from build123d import *

# Parameters (mm, degrees)
EXTRUDE_1_DEPTH     = 4.6
SKETCH_1_R          = 2.625
SKETCH_1_W          = 40.4
SKETCH_1_H          = 4.6
CUT_EXTRUDE_1_DEPTH = 4.6
FILLET_1_R          = 5
FILLET_2_R          = 4


with BuildPart() as part:
    # 草图3 → 凸台-拉伸1 (new body)
    with BuildSketch(Plane(origin=(0, 0, 0), x_dir=(1, 0, 0), z_dir=(0, 1, 0))):
        Polygon((-40, 28), (-60, 28), (-60, -28), (-40, -28), (18.5, -28), (18.5, -36), (45, -36), (45, -28), (45, 28), (45, 36), (18.5, 36), (18.5, 28), align=None)
    extrude(amount=EXTRUDE_1_DEPTH)

    # 草图1 → 切除-拉伸1 (cut)
    with BuildSketch(Plane(origin=(0, 0, 0), x_dir=(1, 0, 0), z_dir=(0, 1, 0))):
        with Locations(Location((-31.75, 20.6375, 0), (0, 0, 270))):
            Circle(SKETCH_1_R)
        with Locations(Location((31.75, 20.6375, 0), (0, 0, 90))):
            Circle(SKETCH_1_R)
        with Locations(Location((31.75, -20.6375, 0), (0, 0, 270))):
            Circle(SKETCH_1_R)
        with Locations(Location((-31.75, -20.6375, 0), (0, 0, 90))):
            Circle(SKETCH_1_R)
        with Locations((-28, -10.4375)):
            Rectangle(SKETCH_1_W, SKETCH_1_H)
        with Locations((-28, 10.4375)):
            Rectangle(SKETCH_1_W, SKETCH_1_H)
        Polygon((-22.25, -26.5375), (-22.25, -14.7375), (-0.65, -14.7375), (-0.65, -26.5375), (-0.65, -30.009482824), (-22.25, -30.009482824), align=None)
        Polygon((-22.25, 14.7375), (-0.65, 14.7375), (-0.65, 26.5375), (-0.65, 30.009482824), (-22.25, 30.009482824), (-22.25, 26.5375), align=None)
    extrude(amount=CUT_EXTRUDE_1_DEPTH, mode=Mode.SUBTRACT)

    # 圆角1
    fillet_1_edges = [part.edges().sort_by_distance(p)[0] for p in [
        (-22.25, 2.3, 14.7375),
        (-0.65, 2.3, 14.7375),
        (-0.65, 2.3, -14.7375),
        (-22.25, 2.3, -14.7375),
    ]]
    fillet(fillet_1_edges, radius=FILLET_1_R)

    # 圆角2
    fillet_2_edges = [part.edges().sort_by_distance(p)[0] for p in [
        (-0.65, 2.3, 28),
        (-22.25, 2.3, 28),
        (-0.65, 2.3, -28),
        (-22.25, 2.3, -28),
        (-60, 2.3, 28),
        (-60, 2.3, -28),
        (18.5, 2.3, -28),
        (18.5, 2.3, -36),
        (45, 2.3, -36),
        (45, 2.3, 36),
        (18.5, 2.3, 36),
        (18.5, 2.3, 28),
    ]]
    fillet(fillet_2_edges, radius=FILLET_2_R - 0.0001)  # a hair under: the kernel refuses the full size


solid = part.part
Model file for the job. Use its own axes, mm. A direction names the side the tool comes from. Round coordinates to 2 decimals unless told otherwise and drop trailing zeros. Order: outer loops, then holes, each group sorted by start corner. A loop starts at its lowest first (then second) coordinate and runs counter-clockwise, first axis right, second up.
(1) 3-axis set-ups, long thin cutter, end or side, ignore diameter. For faces 1 (the face through (32, 2, -36)), 2 (the face through (-41, 2, -28)), 3 (the face through (-22.25, 2, -22)), 4 (the face through (-23.453, 2.268, 26.859)), 5 (the face through (-7.8, 2, 10)): which of +Z, -Z, +X, -X, +Y, -Y reach the whole face in a straight line?
(2) Band-saw the part on A-A (x = -36.5). List the corners of the cut face in (y, z).
(3) Pin check, flat tips, straight feed: pin 1 (1.4 mm diameter, centred on x = -13.5, y = 3, fed in from -Z); pin 2 (3 mm diameter, centred on x = -31.75, z = -20.64, fed in from +Y); pin 3 (1.5 mm diameter, centred on x = -31, y = 1.5, fed in from -Z); pin 4 (1.4 mm diameter, centred on x = -20, y = 2, fed in from +Z). Stop position of each tip, or through.
(4) Band-saw the part on B-B (z = -16.5). List the corners of the cut face in (x, y).
(5) Band-saw the part on D-D (y = 3.4). Give the number of separate pieces and of enclosed holes in the cut face, then the cut area to 3 significant figures.
(6) Drill centre lines: line 1 (Z direction, x = -43, y = 4.2); line 2 (X direction, y = 2.7, z = 9); line 3 (X direction, y = 3.4, z = -22). Where is each one in solid material? Low to high.
(7) Pull direction Z, two halves, no side cores. Call faces 6 (the face through (-2.076, 2.332, 16.241)), 7 (the face through (-28, 2, 8.137)), 8 (the face through (-2.154, 2.332, -16.163)): released by +Z, released by -Z, zero draft, split by the parting line, or undercut.
(8) Band-saw the part on C-C (x = 31.75). List the corners of the cut face in (y, z).
Verdict:
1. face 1: -Z, +X, -X, +Y, -Y
1. face 2: -Z, -X, +Y, -Y
1. face 3: -Z, +Y, -Y
1. face 4: +Z, +Y, -Y
1. face 5: +Y, -Y
2. outline: (0, -28) - (4.6, -28) - (4.6, -12.74) - (0, -12.74) - close; (0, -8.14) - (4.6, -8.14) - (4.6, 8.14) - (0, 8.14) - close; (0, 12.74) - (4.6, 12.74) - (4.6, 28) - (0, 28) - close
3. pin 1: stops at z = -14.74
3. pin 2: passes through
3. pin 3: stops at z = -28
3. pin 4: stops at z = 16.12
4. outline: (-60, 0) - (-21.06, 0) - (-21.06, 4.6) - (-60, 4.6) - close; (-1.84, 0) - (45, 0) - (45, 4.6) - (-1.84, 4.6) - close
5. separate pieces: 1
5. enclosed holes: 6
5. area: 5,270 mm2
6. line 1: z = -28 to -12.74, -8.14 to 8.14, 12.74 to 28
6. line 2: x = -60 to -48.2, -7.8 to 45
6. line 3: x = -60 to -33.99, -29.51 to -22.25, -0.65 to 29.51, 33.99 to 45
7. face 6: released by +Z
7. face 7: undercut
7. face 8: released by -Z
8. outline: (0, -36) - (4.6, -36) - (4.6, -23.26) - (0, -23.26) - close; (0, -18.01) - (4.6, -18.01) - (4.6, 18.01) - (0, 18.01) - close; (0, 23.26) - (4.6, 23.26) - (4.6, 36) - (0, 36) - close
